For this review, use the dimensioned drawing (mm, ordinates from the lowest corner) and the shaded views. A direction names the side the tool comes from. Give positions to 0.01 mm unless a question says otherwise; leave off trailing zeros. Order: outer loops, then holes, each group sorted by start corner. A loop starts at its lowest first (then second) coordinate and runs counter-clockwise, first axis right, second up.
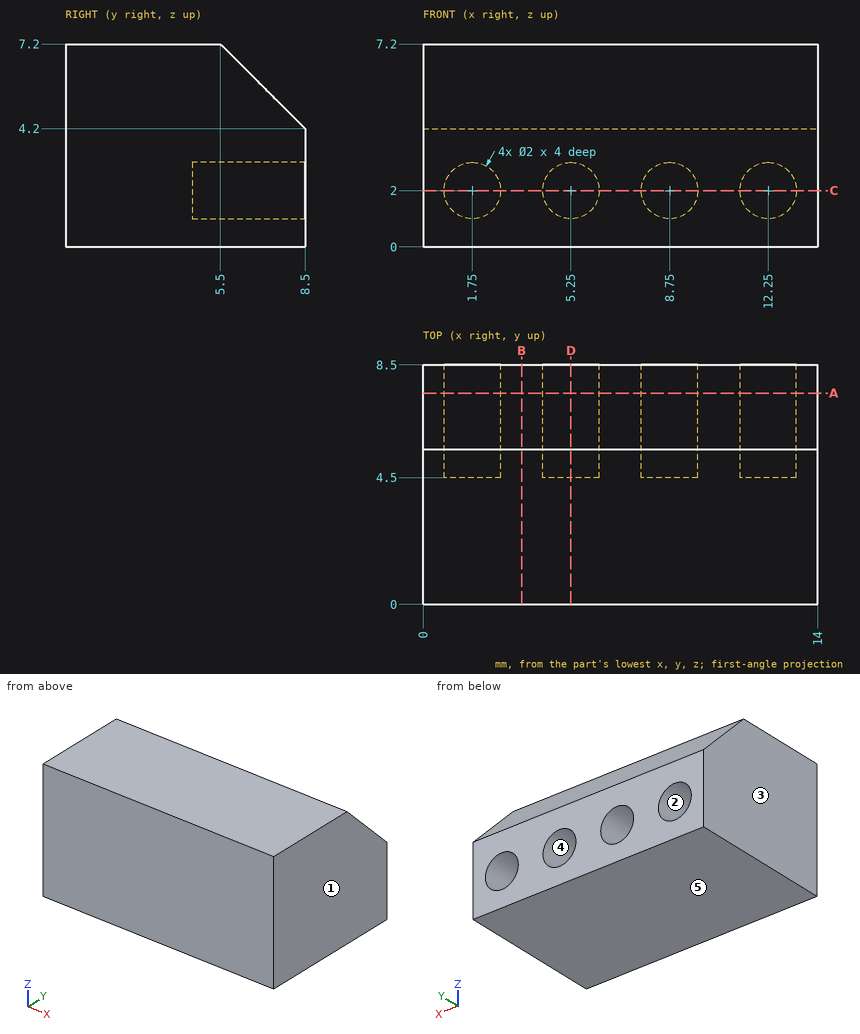
1. Take a section at A-A (y = 7.5). State the section outline as (x, z) points.
Recorded:
outline: (0, 0) - (14, 0) - (14, 5.2) - (0, 5.2) - close; hole circle Ø2 at (1.75, 2); hole circle Ø2 at (5.25, 2); hole circle Ø2 at (8.75, 2); hole circle Ø2 at (12.25, 2)
2. Take a section at D-D (x = 5.25). State the section outline as (y, z) points, then the cut area to 3 significant figures.
Recorded:
outline: (0, 0) - (8.5, 0) - (8.5, 1) - (4.5, 1) - (4.5, 3) - (8.5, 3) - (8.5, 4.2) - (5.5, 7.2) - (0, 7.2) - close
area: 48.7 mm2
3. Draft analysis for pull direction X (two halves, no side actions). For the marked faces 3, 4 and 5, state which applies: pulls with the +X half, pulls with the -X half, needs draft (parallel to the pull), parting line crosses it, or undercut.
Recorded:
face 3: pulls with the -X half
face 4: undercut
face 5: needs draft
4. Take a section at B-B (x = 3.5). State the section outline as (y, z) points.
Recorded:
outline: (0, 0) - (8.5, 0) - (8.5, 4.2) - (5.5, 7.2) - (0, 7.2) - close
5. Take a section at C-C (z = 2). State the section outline as (x, y) points.
Recorded:
outline: (0, 0) - (14, 0) - (14, 8.5) - (13.25, 8.5) - (13.25, 4.5) - (11.25, 4.5) - (11.25, 8.5) - (9.75, 8.5) - (9.75, 4.5) - (7.75, 4.5) - (7.75, 8.5) - (6.25, 8.5) - (6.25, 4.5) - (4.25, 4.5) - (4.25, 8.5) - (2.75, 8.5) - (2.75, 4.5) - (0.75, 4.5) - (0.75, 8.5) - (0, 8.5) - close
6. For line 1 along X through (y, z) = (5.5, 2); line 2 along Y through (x, z) = (8.75, 1.5); line 3 along Z through (x, y) = (9, 6), list the stretches that pass through material, from the lowest coordinate up.
Recorded:
line 1: x = 0 to 0.75, 2.75 to 4.25, 6.25 to 7.75, 9.75 to 11.25, 13.25 to 14
line 2: y = 0 to 4.5
line 3: z = 0 to 1.03, 2.97 to 6.7
7. Machinability: for the marked faces 1 and 2, which of the approach directions +Z, -Z, +X, -X, +Y, -Y give a long, thin tool a straight path to every point of the face, cutting with its end or side? Answer none if there is none.
Recorded:
face 1: +Z, -Z, +X, +Y, -Y
face 2: +Y
